Work out the finished part from the listing and answer in its coordinate system (mm). Give positions to 0.01 mm unless a question says otherwise; leave off trailing zeros. Write each loop counter-clockwise with the first axis right and the second up, starting at its lowest first coordinate (ties: lowest second). Pieces come first, ordered by that corner, then holes. Notation, with made-up numbers: (-15, -19.75) - (5, -19.75) arc R20 cw to (5, 2.25) - close; hole circle Ø10 at (-29, -2). An arc over 180 degrees is marked (long way). Write item = value, one per line.
from build123d import *

# Parameters (mm, degrees)
SKETCH1_R           = 3
SKETCH1_R_2         = 22.6
BOSS_EXTRUDE1_DEPTH = 4
CUT_EXTRUDE1_DEPTH  = 5
SKETCH3_R           = 3.15
BOSS_EXTRUDE2_DEPTH = 4
FILLET1_R           = 5
SKETCH4_R           = 1.5
CUT_EXTRUDE2_DEPTH  = 5


with BuildPart() as part:
    # Sketch1 → Boss-Extrude1 (new body)
    with BuildSketch(Plane.XY):
        Polygon((0, 36.632796194), (-7.647271147, 32.990762303), (-9.405300929, 29.104152359), (-58.126981429, 27.62278105), (-76.5, 14.085859857), (-76.5, -14.085859857), (-58.126981429, -27.62278105), (-9.405300929, -29.104152359), (-7.647271147, -32.990762303), (0, -36.632796194), (7.647271147, -32.990762303), (9.405300929, -29.104152359), (58.126981429, -27.62278105), (76.5, -14.085859857), (76.5, 14.085859857), (58.126981429, 27.62278105), (9.405300929, 29.104152359), (7.647271147, 32.990762303), align=None)
        with Locations((0, 30)):
            Circle(SKETCH1_R, mode=Mode.SUBTRACT)
        with Locations((-50, 0)):
            Circle(SKETCH1_R_2, mode=Mode.SUBTRACT)
        with Locations((50, 0)):
            Circle(SKETCH1_R_2, mode=Mode.SUBTRACT)
        with Locations((0, -30)):
            Circle(SKETCH1_R, mode=Mode.SUBTRACT)
    extrude(amount=BOSS_EXTRUDE1_DEPTH)

    # Sketch2 → Cut-Extrude1 (cut, through all)
    with BuildSketch(Plane.XY.offset(4)):
        with BuildLine():
            Line((8.5, 20), (-8.5, 20))
            ThreePointArc((-8.5, 20), (-11.328427125, 18.828427125), (-12.5, 16))
            Line((-12.5, 16), (-12.5, -16))
            ThreePointArc((-12.5, -16), (-11.328427125, -18.828427125), (-8.5, -20))
            Line((-8.5, -20), (8.5, -20))
            ThreePointArc((8.5, -20), (11.328427125, -18.828427125), (12.5, -16))
            Line((12.5, -16), (12.5, 16))
            ThreePointArc((12.5, 16), (11.328427125, 18.828427125), (8.5, 20))
        make_face()
    extrude(amount=-CUT_EXTRUDE1_DEPTH, mode=Mode.SUBTRACT)

    # Sketch3 → Boss-Extrude2 (add)
    with BuildSketch(Plane.XY.offset(4)):
        Polygon((-58.126981429, 27.62278105), (-64.551915182, 31.10998542), (-77.245081729, 28.773819798), (-73.717039059, 16.136297176), align=None)
        with Locations((-70, 25)):
            Circle(SKETCH3_R, mode=Mode.SUBTRACT)
        Polygon((73.717039059, 16.136297176), (58.126981429, 27.62278105), (64.551915182, 31.10998542), (77.245081729, 28.773819798), align=None)
        with Locations((70, 25)):
            Circle(SKETCH3_R, mode=Mode.SUBTRACT)
        Polygon((58.126981429, -27.62278105), (64.551915182, -31.10998542), (77.245081729, -28.773819798), (73.717039059, -16.136297176), align=None)
        with Locations((70, -25)):
            Circle(SKETCH3_R, mode=Mode.SUBTRACT)
        Polygon((-73.717039059, -16.136297176), (-58.126981429, -27.62278105), (-64.551915182, -31.10998542), (-77.245081729, -28.773819798), align=None)
        with Locations((-70, -25)):
            Circle(SKETCH3_R, mode=Mode.SUBTRACT)
    extrude(amount=-BOSS_EXTRUDE2_DEPTH)

    # Fillet1
    fillet1_edges = [part.edges().sort_by_distance(p)[0] for p in [
        (77.245081729, 28.773819798, 2),
        (77.245081729, -28.773819798, 2),
        (-77.245081729, -28.773819798, 2),
        (-77.245081729, 28.773819798, 2),
    ]]
    fillet(fillet1_edges, radius=FILLET1_R)

    # Sketch4 → Cut-Extrude2 (cut, through all)
    with BuildSketch(Plane.XY.offset(4)):
        with Locations((-50, 23.75)):
            Circle(SKETCH4_R)
        with Locations((-70.56810334, 11.875)):
            Circle(SKETCH4_R)
        with Locations((-70.56810334, -11.875)):
            Circle(SKETCH4_R)
        with Locations((-50, -23.75)):
            Circle(SKETCH4_R)
        with Locations((-29.43189666, -11.875)):
            Circle(SKETCH4_R)
        with Locations((-29.43189666, 11.875)):
            Circle(SKETCH4_R)
        with Locations((29.43189666, 11.875)):
            Circle(SKETCH4_R)
        with Locations((29.43189666, -11.875)):
            Circle(SKETCH4_R)
        with Locations((50, -23.75)):
            Circle(SKETCH4_R)
        with Locations((70.56810334, -11.875)):
            Circle(SKETCH4_R)
        with Locations((70.56810334, 11.875)):
            Circle(SKETCH4_R)
        with Locations((50, 23.75)):
            Circle(SKETCH4_R)
    extrude(amount=-CUT_EXTRUDE2_DEPTH, mode=Mode.SUBTRACT)


solid = part.part
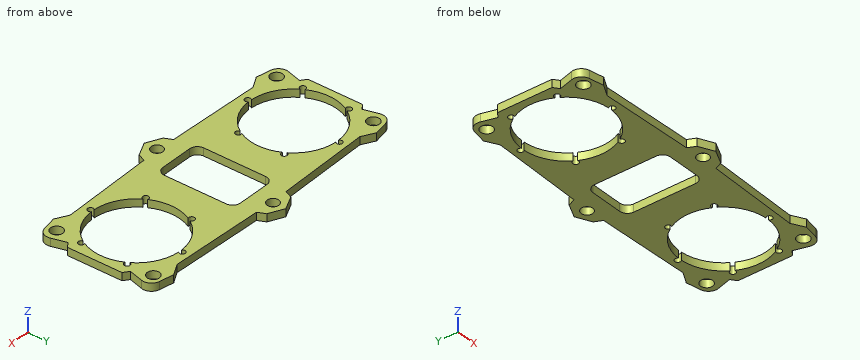
1. Find section B-B, the plane y = 8.5. Give the vertices of the cut face in (x, z).
Solution:
outline = (-76.5, 0) - (-70.94, 0) - (-70.94, 4) - (-76.5, 4) - close; (-29.06, 0) - (-12.5, 0) - (-12.5, 4) - (-29.06, 4) - close; (12.5, 0) - (29.06, 0) - (29.06, 4) - (12.5, 4) - close; (70.94, 0) - (76.5, 0) - (76.5, 4) - (70.94, 4) - close
2. Given pin 1 (2 mm diameter, centred on x = -23.5, z = 1.5, fed in from +Y); pin 2 (2 mm diameter, centred on x = -39.5, z = 1, fed in from +Y); pin 3 (1.2 mm diameter, centred on x = 2, z = 3, fed in from -Y), each flat-ended and moving along its own axis, determine where each tip first touches the part or whether it passes through.
Solution:
pin_1 = 28.71
pin_2 = 28.22
pin_3 = -35.97
3. Find section C-C, the plane z = 0.7. Give the number of separate pieces and of enclosed holes in the cut face, then the cut area to 3 significant figures.
Solution:
separate_pieces = 1
enclosed_holes = 9
area = 4,450 mm^2
4. Find section D-D, the plane x = 24.5. Give the vertices of the cut face in (y, z), then the cut area to 3 significant figures.
Solution:
outline = (-28.65, 0) - (28.65, 0) - (28.65, 4) - (-28.65, 4) - close
area = 229 mm^2
5. Find section A-A, the plane x = -62. Give the vertices of the cut face in (y, z), then the cut area to 3 significant figures.
Solution:
outline = (-29.72, 0) - (-19.15, 0) - (-19.15, 4) - (-29.72, 4) - close; (19.15, 0) - (29.72, 0) - (29.72, 4) - (19.15, 4) - close
area = 84.6 mm^2
6. Straight lines are drawn through the part: line 1 (X direction, y = -0.5, z = 1.05); line 2 (X direction, y = 12, z = 0.4); line 3 (Y direction, x = 0, z = 2). For each, find the intervals that lie inside material, in ascending order.
Solution:
line_1 = -76.5 to -72.59, -27.41 to -12.5, 12.5 to 27.41, 72.59 to 76.5
line_2 = -76.5 to -72.06, -27.94 to -12.5, 12.5 to 27.94, 72.06 to 76.5
line_3 = -36.63 to -33, -27 to -20, 20 to 27, 33 to 36.63
